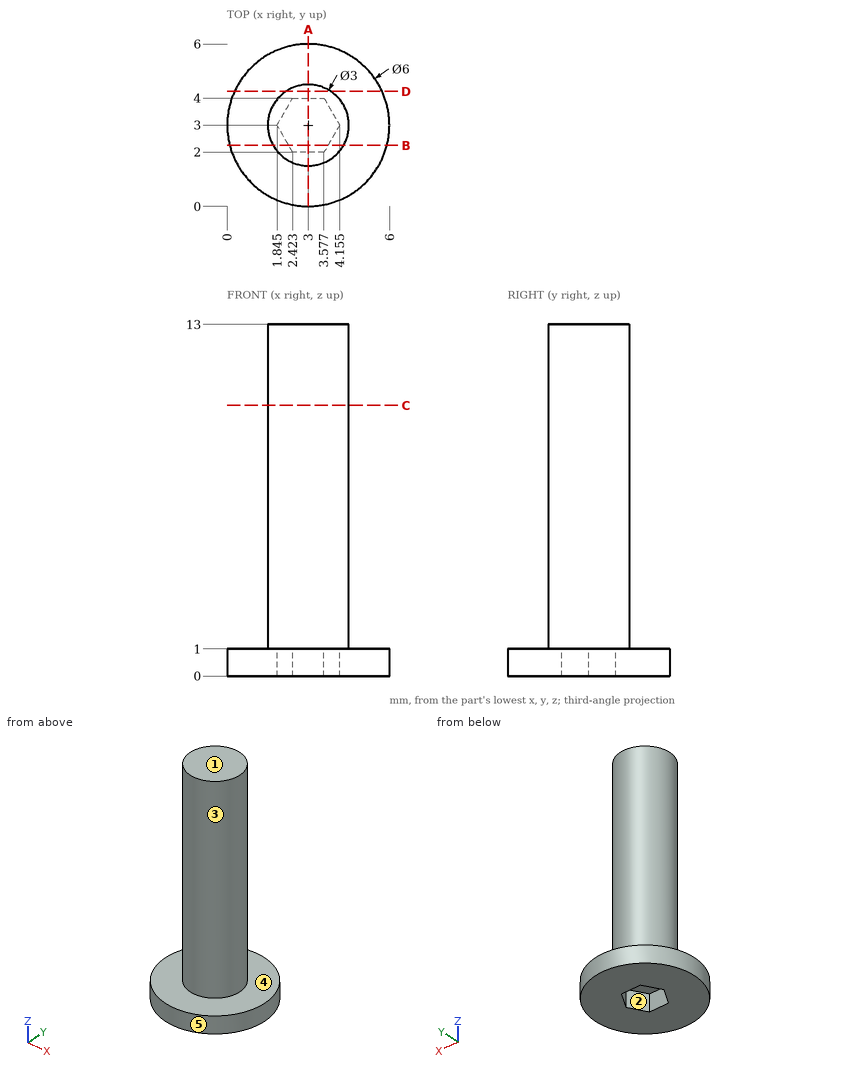
Input: dimensioned drawing with shaded views. Units: mm. Origin: part minimum x, y, z. A direction names the side the tool comes from. Coordinates: 2 decimals unless noted, no trailing zeros. Loops run counter-clockwise (first coordinate to the right, second up) from the corner with the lowest first, then second, coordinate; pieces in that order, holes last. Notation, with made-up numbers: M 78.25,-0.5 L 120.25,-0.5 A30 ccw 120.25,34.5 Z; hole C 78,65.25 d8. An arc over 180 degrees is marked long. One line per item, written item: value. Start each with the question number.
1) Cut plane C-C (z = 10). Return loops of the section in (x, y).
2) Cut plane D-D (y = 4.25). Return loops of the section in (x, z).
3) Draft query along Y for the marked faces 1, 2 and 3. Return one class per face: released by +Y, released by -Y, zero draft, split by the parting line, or undercut.
4) Cut plane B-B (y = 2.25). Return loops of the section in (x, z) (1 decimal).
5) Pin query (flat end, axial travel): P1, Ø2, axis at x = 1, z = 7.5, coming from the +Y side; P2, Ø3, axis at x = 4.5, z = 4.5, coming from the -Y side; P3, Ø1.6, axis at x = 3, y = 3, coming from the -Z side. Return the tip coordinate at first contact, or that it passes through.
6) Cut plane A-A (x = 3). Return loops of the section in (y, z), then the cut area to 3 significant figures.
7) Reachability of the marked faces 4 and 5 from +Z, -Z, +X, -X, +Y, -Y: full face, straight path, thin tool, end or side. Return the list, or none.
8) Material intervals for L1, parallel to Z at x = 1.05, y = 4.9; L2, parallel to Y at x = 5.25, z = 0.5 (1 decimal); L3, parallel to X at y = 2.5, z = 4 (1 decimal), sorted ascending. Write a range as from..to.
Evaluation:
1. outline: C 3,3 d3
2. outline: M 0.27,0 L 5.73,0 L 5.73,1 L 3.83,1 L 3.83,13 L 2.17,13 L 2.17,1 L 0.27,1 Z
3. face 1: zero draft
3. face 2: undercut
3. face 3: split by the parting line
4. outline: M 0.1,0 L 2.3,0 L 2.3,1 L 3.7,1 L 3.7,0 L 5.9,0 L 5.9,1 L 4.3,1 L 4.3,13 L 1.7,13 L 1.7,1 L 0.1,1 Z
5. P1: y = 4.12
5. P2: y = 1.5
5. P3: z = 1
6. outline: M 0,0 L 2,0 L 2,1 L 4,1 L 4,0 L 6,0 L 6,1 L 4.5,1 L 4.5,13 L 1.5,13 L 1.5,1 L 0,1 Z
6. area: 40.0 mm^2
7. face 4: +Z
7. face 5: +Z, -Z
8. L1: 0..1
8. L2: 1..5
8. L3: 1.6..4.4
